from build123d import *

# Parameters (mm, degrees)
BOSS_EXTRUDE1_DEPTH  = 270
FILLET1_R            = 2
CUT_EXTRUDE1_DEPTH   = 5
FILLET1_OF_MIRROR1_R = 2
FILLET2_R            = 3


with BuildPart() as part:
    # Sketch1 → Boss-Extrude1 (new, symmetric)
    with BuildSketch(Plane(origin=(0, 0, 0), x_dir=(0, 0, -1), z_dir=(1, 0, 0))):
        Polygon((23.094010768, 0), (11.547005384, 20), (-11.547005384, 20), (-23.094010768, 0), (-11.547005384, -20), (11.547005384, -20), align=None)
    extrude(amount=BOSS_EXTRUDE1_DEPTH, both=True)

    # Sketch2 → Revolve1 (revolve)
    with BuildSketch(Plane.XY):
        Polygon((270, 17.5), (300, 17.5), (300, 15), (350, 15), (350, 14), (395, 14), (395, 0), (270, 0), align=None)
    revolve1 = revolve(axis=Axis((395, 0, 0), (-1, 0, 0)))

    # Fillet1
    # the kernel refuses this fillet: 2 mm, written as the material it adds along each edge
    with BuildSketch(Plane(origin=(300, 0, 0), x_dir=(0, 1, 0), z_dir=(0, 0, 1))) as fillet1_piece_1:
        with BuildLine():
            CenterArc((15 + FILLET1_R, -FILLET1_R), FILLET1_R, 90, 90)
            Line((15, -FILLET1_R), (15 - FILLET1_R * 0.02, -FILLET1_R))
            Line((15 - FILLET1_R * 0.02, -FILLET1_R), (15 - FILLET1_R * 0.02, FILLET1_R * 0.02))
            Line((15 - FILLET1_R * 0.02, FILLET1_R * 0.02), (15 + FILLET1_R, FILLET1_R * 0.02))
            Line((15 + FILLET1_R, FILLET1_R * 0.02), (15 + FILLET1_R, 0))
        make_face()
    revolve(axis=Axis((300, 0, 0), (-1, 0, 0)))
    with BuildSketch(Plane(origin=(350, 0, 0), x_dir=(0, 1, 0), z_dir=(0, 0, 1))) as fillet1_piece_2:
        with BuildLine():
            CenterArc((16, -1.732050808), FILLET1_R, 120, 60)
            Line((14, -1.732050808), (13.96, -1.732050808))
            Line((13.96, -1.732050808), (13.96, 0))
            Line((13.96, 0), (14, 0.04))
            ThreePointArc((14, 0.04), (14.5, 0.04), (14.98, 0.034641016))
            Line((14.98, 0.034641016), (15, 0))
        make_face()
    revolve(axis=Axis((350, 0, 0), (-1, 0, 0)))

    # Sketch3 → Cut-Extrude1 (cut)
    with BuildSketch(Plane(origin=(0, 15, 0), x_dir=(1, 0, 0), z_dir=(0, 1, 0))):
        with BuildLine():
            Line((307, 5), (343, 5))
            ThreePointArc((343, 5), (348, 0), (343, -5))
            Line((343, -5), (307, -5))
            ThreePointArc((307, -5), (302, 0), (307, 5))
        make_face()
    cut_extrude1 = extrude(amount=-CUT_EXTRUDE1_DEPTH, mode=Mode.SUBTRACT)

    # Mirror1: Revolve1, Cut-Extrude1 across plane
    add(revolve1.mirror(Plane(origin=(0, 0, 0), x_dir=(0, 0, 1), z_dir=(1, 0, 0))))
    add(cut_extrude1.mirror(Plane(origin=(0, 0, 0), x_dir=(0, 0, 1), z_dir=(1, 0, 0))), mode=Mode.SUBTRACT)

    # Fillet1 of Mirror1
    # the kernel refuses this fillet: 2 mm, written as the material it adds along each edge
    with BuildSketch(Plane(origin=(-300, 0, 0), x_dir=(0, 1, 0), z_dir=(0, 0, 1))) as fillet1_of_mirror1_piece_1:
        with BuildLine():
            CenterArc((15 + FILLET1_OF_MIRROR1_R, FILLET1_OF_MIRROR1_R), FILLET1_OF_MIRROR1_R, 180, 90)
            Line((15, FILLET1_OF_MIRROR1_R), (15 - FILLET1_OF_MIRROR1_R * 0.02, FILLET1_OF_MIRROR1_R))
            Line((15 - FILLET1_OF_MIRROR1_R * 0.02, FILLET1_OF_MIRROR1_R), (15 - FILLET1_OF_MIRROR1_R * 0.02, -FILLET1_OF_MIRROR1_R * 0.02))
            Line((15 - FILLET1_OF_MIRROR1_R * 0.02, -FILLET1_OF_MIRROR1_R * 0.02), (15 + FILLET1_OF_MIRROR1_R, -FILLET1_OF_MIRROR1_R * 0.02))
            Line((15 + FILLET1_OF_MIRROR1_R, -FILLET1_OF_MIRROR1_R * 0.02), (15 + FILLET1_OF_MIRROR1_R, 0))
        make_face()
    revolve(axis=Axis((-300, 0, 0), (-1, 0, 0)))
    with BuildSketch(Plane(origin=(-350, 0, 0), x_dir=(0, 1, 0), z_dir=(0, 0, 1))) as fillet1_of_mirror1_piece_2:
        with BuildLine():
            CenterArc((16, 1.732050808), FILLET1_OF_MIRROR1_R, 180, 60)
            Line((14, 1.732050808), (13.96, 1.732050808))
            Line((13.96, 1.732050808), (13.96, 0))
            Line((13.96, 0), (14, -0.04))
            ThreePointArc((14, -0.04), (14.5, -0.04), (14.98, -0.034641016))
            Line((14.98, -0.034641016), (15, 0))
        make_face()
    revolve(axis=Axis((-350, 0, 0), (-1, 0, 0)))

    # Fillet2
    fillet2_edges = [part.edges().sort_by_distance(p)[0] for p in [
        (0, -20, -11.547005384),
        (0, -20, 11.547005384),
        (0, 0, 23.094010768),
        (0, 20, 11.547005384),
        (0, 20, -11.547005384),
        (0, 0, -23.094010768),
    ]]
    fillet(fillet2_edges, radius=FILLET2_R)

    # Sketch5 → Tap Drill for M8 Tap1 (revolve, cut)
    with BuildSketch(Plane(origin=(395, 0, 0), x_dir=(0, 0, -1), z_dir=(0, 1, 0))):
        Polygon((0, 0), (0, 27.5), (3.4, 25.457073895), (3.4, 0.025), (3.425, 0), align=None)
    tap_drill_for_m8_tap1 = revolve(axis=Axis((401.35, 0, 0), (-1, 0, 0)), mode=Mode.SUBTRACT)

    # Mirror2: Tap Drill for M8 Tap1 across plane
    add(tap_drill_for_m8_tap1.mirror(Plane(origin=(0, 0, 0), x_dir=(0, 0, 1), z_dir=(1, 0, 0))), mode=Mode.SUBTRACT)


solid = part.part
The listing builds one solid part. Answer for the finished solid, in the listing's coordinates (mm). A direction names the side the tool comes from. Give positions to 0.01 mm unless a question says otherwise; leave off trailing zeros. Write each loop counter-clockwise with the first axis right and the second up, starting at its lowest first coordinate (ties: lowest second). Pieces come first, ordered by that corner, then holes.
Item 1: Section A-A, the plane x = 42.5 is taken. Write down the section's boundary in (y, z), plus the area to 3 significant figures.
Item 2: Find the intervals of material crossed by line 1 along Y through (x, z) = (379.75, 0); line 2 along X through (y, z) = (18.5, 4.5), in increasing order.
Item 3: Flat-ended cylindrical pins translate along their axes: P1, Ø6, axis at y = 0, z = 0, coming from the +X side; P2, Ø4, axis at x = -51, y = 3.5, coming from the +Z side; P3, Ø5.5, axis at y = 0, z = 0, coming from the +X side. Find the tip coordinate at first contact, or state that the pin passes through.
Item 4: Which of the six approach directions +Z, -Z, +X, -X, +Y, -Y give full straight-line access (tool end or side, diameter ignored) to faces 1 (the flat face through (-270, 9, 15.2)), 2 (the flat face through (300, -3, -17)), 3 (the flat face through (4, 20, 0))?
Completed:
1. outline: (-20, -9.81) arc R3 ccw to (-18.5, -12.41) - (-1.5, -22.23) arc R3 ccw to (1.5, -22.23) - (18.5, -12.41) arc R3 ccw to (20, -9.81) - (20, 9.81) arc R3 ccw to (18.5, 12.41) - (1.5, 22.23) arc R3 ccw to (-1.5, 22.23) - (-18.5, 12.41) arc R3 ccw to (-20, 9.81) - close
1. area: 1,380 mm2
2. line 1: y = -14 to -3.4, 3.4 to 14
2. line 2: x = -270 to 270
3. P1: stops at x = 369.3
3. P2: stops at z = 22.23
3. P3: stops at x = 369.15
4. face 1: -X
4. face 2: +X
4. face 3: +Z, -Z, +X, -X, +Y
